Model file for the job. Use its own axes, mm. Face numbers are marked on the shaded views. A direction names the side the tool comes from. Give positions to 0.01 mm unless a question says otherwise; leave off trailing zeros. Write each loop counter-clockwise with the first axis right and the second up, starting at its lowest first coordinate (ties: lowest second). Pieces come first, ordered by that corner, then holes. Notation, with made-up numbers: M 42.25,65 L 63.25,65 A5 ccw 63.25,73 Z; hole C 15,23 d2. An arc over 180 degrees is marked long. Answer as a JSON object with one key per item and string values. Group by question number.
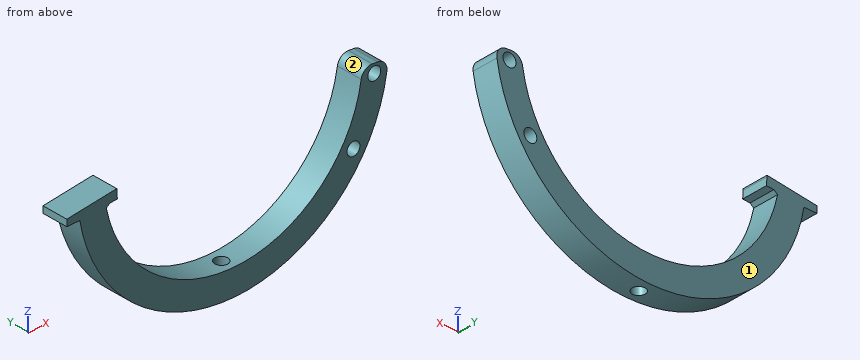
Autodesk Inventor part; units mm, degrees
ref_plane "YZ Plane" through (0, 0, 0) normal (1, 0, 0) x (0, 1, 0)
ref_plane "XZ Plane" through (0, 0, 0) normal (0, 1, 0) x (-1, 0, 0)
ref_plane "XY Plane" through (0, 0, 0) normal (0, 0, 1) x (1, 0, 0)
sketch "Schizzo1" plane through (0, 0, 0) normal (0, 1, 0) x (-1, 0, 0)
  arc A0 (-49.8426, -3.9646) -> (48.9431, -10.2263) centre (0, 0) ccw
  arc A1 (-59.8111, -4.7575) -> (59.1221, -10.2263) centre (0, 0) ccw
  circle A2 centre (-54.4546, -7.7263) radius 2.5
  line L0 (-49.8426, -3.9646) -> (-59.8111, -4.7575)
  line L1 (59.1221, -10.2263) -> (64.1458, -10.2263)
  line L2 (64.1458, -10.2263) -> (64.1458, -7.7263)
  line L3 (64.1458, -10.2263) -> (44.6472, -8.9763)
  line L4 (48.9431, -10.2263) -> (47.4892, -9.1585)
  line L5 (44.8385, -5.9924) -> (44.6472, -8.9763)
  line L6 (64.1458, -7.7263) -> (44.8741, -5.4367)
  line L7 (44.8741, -5.4367) -> (44.8385, -5.9924)
  dimension "d0" = 100
  dimension "d6" = 5
  dimension "d8" = 2.5
  dimension "d9" = 2.5
extrude "Estrusione1" add sketch "Schizzo1" along normal mid plane 10 contours A0 L4 L3 L1 A1 L0 | L3 L5 L7 L6 L2 | A2
extrude "Estrusione2" cut sketch "Schizzo1" along normal through all both and the other way through all contours A2
fillet "Raccordo3" radius 4 1 edges at (59.8111, 0, -4.7575)
fillet "Raccordo4" radius 4 1 edges at (49.8426, 0, -3.9646)
sketch "Schizzo2" plane through (0, 5, 0) normal (0, 1, 0) x (1, 0, 0)
  circle A0 centre (46.4198, 29.499) radius 2.5
  circle A1 centre (54.4546, 7.7263) radius 2.5
  arc A2 (49.412, 7.6457) -> (-48.9431, 10.2263) centre (0, 0) ccw
  line L0 (42.1413, 26.9094) -> (50.6984, 32.0886) construction
  arc A3 (59.3185, 9.0175) -> (-59.1221, 10.2263) centre (0, 0) ccw
  point P0 (-49.51, 6.9828)
  point P1 (-59.5579, 7.2704)
  point P2 (-60, 0)
  point P3 (-50, 0)
  dimension "d19" = 29.499
  dimension "d20" = 24.2008
extrude "Estrusione3" cut sketch "Schizzo2" against normal blind 10 contours A0
sketch "Schizzo4" plane through (0, 0, 0) normal (0, 0, 1) x (1, 0, 0)
  circle A0 centre (0, 0) radius 2.5
  dimension "d28" = 5
extrude "Estrusione5" cut sketch "Schizzo4" against normal through all
properties part number "ganascia"
Q1. Drop flat-ended pins along their axis: P1, Ø2, axis at x = -31, y = -2, coming from the +Z side; P2, Ø5, axis at y = 1.5, z = -48, coming from the -X side; P3, Ø2.5, axis at x = -61, y = 0, coming from the -Z side; P4, Ø3, axis at x = 54.45, z = -7.73, coming from the +Y side. Give the stop position or say it passes through.
Q2. Slice it at A-A, the plane x = 0. Write the cut outline in (y, z).
Q3. Slice it at B-B, the plane y = 0. Write the cut outline in (x, z), then the cut area to 3 significant figures.
Q4. Wall check: L1, parallel to Y at x = 0, z = -54; L2, parallel to X at y = -2.75, z = -29; L3, parallel to X at y = -2.75, z = -30. Give the ranges that are in metal, low to high.
Q5. Slice it at D-D, the plane x = -33.5. Write the cut outline in (y, z).
Q6. 3-axis set-ups, long thin cutter, end or side, ignore diameter. For the marked faces 1 and 2: which of +Z, -Z, +X, -X, +Y, -Y reach the whole face in a straight line?
Q7. Slice it at C-C, the plane z = -15.5. Write the cut outline in (x, y), then the cut area to 3 significant figures.
Solved:
{
 "1": {"P1": "stops at z = -38.42", "P2": "stops at x = -39.11", "P3": "stops at z = -10.23", "P4": "passes through"},
 "2": {"outline": "M -5,-60 L -2.5,-60 L -2.5,-50 L -5,-50 Z; M 2.5,-60 L 5,-60 L 5,-50 L 2.5,-50 Z"},
 "3": {"outline": "M -64.15,-10.23 L -59.12,-10.23 A60 ccw -2.5,-59.95 L -2.5,-49.94 A50 cw -48.94,-10.23 L -47.49,-9.16 L -44.65,-8.98 L -44.84,-5.99 L -44.87,-5.44 L -64.15,-7.73 Z; M 2.5,-59.95 A60 ccw 59.32,-9.02 A4 ccw 55.68,-4.43 L 53.68,-4.27 A4 ccw 49.41,-7.65 A50 cw 2.5,-49.94 Z; hole C 46.42,-29.5 d5; hole C 54.45,-7.73 d5", "area": "1,550 mm²"},
 "4": {"L1": "y = -5 to -2.5, 2.5 to 5", "L2": "x = -52.53 to -40.73, 40.73 to 43.97, 48.87 to 52.53", "L3": "x = -51.96 to -40, 40 to 43.97, 48.87 to 51.96"},
 "5": {"outline": "M -5,-49.78 L 5,-49.78 L 5,-37.12 L -5,-37.12 Z"},
 "6": {"face 1": "+Z, -Z, +X, -X, +Y", "face 2": "+Z, +Y, -Y"},
 "7": {"outline": "M -57.96,-5 L -47.54,-5 L -47.54,5 L -57.96,5 Z; M 47.54,-5 L 57.96,-5 L 57.96,5 L 47.54,5 Z", "area": "209 mm²"}
}
